Could you check a few things on this model? Use its own coordinates, in mm. A direction names the side the tool comes from. Coordinates: 2 decimals unless noted, no trailing zeros. Loops run counter-clockwise (first coordinate to the right, second up) from the corner with the lowest first, then second, coordinate; pieces in that order, holes last. Notation, with made-up numbers: M -1,61 L 54,61 A10 cw 54,72 Z; hole C 11,71 d2. An arc over 180 degrees is marked long. Write each question's results on one line, items separated by ' | '.
```python
from build123d import *

# Parameters (mm, degrees)
F0_W     = 495.3
F0_H     = 495.3
F1_DEPTH = 838.2
F3_DEPTH = 38.1
F5_DEPTH = 38.1
F7_DEPTH = 1117.6
F9_DEPTH = 127


with BuildPart() as f1:
    # F0 (on Top) → F1 (new body)
    with BuildSketch(Plane.XY):
        Rectangle(F0_W, F0_H)
    extrude(amount=F1_DEPTH)

    # F2 (on face) → F3 (join)
    with BuildSketch(Plane.XZ.offset(247.65)):
        with BuildLine():
            ThreePointArc((0, 273.05), (-68.2625, 204.7875), (0, 136.525))
            Line((0, 136.525), (0, 273.05))
        make_face()
        with BuildLine():
            Line((0, 273.05), (0, 136.525))
            ThreePointArc((0, 136.525), (48.268877, 156.518623), (68.2625, 204.7875))
            ThreePointArc((68.2625, 204.7875), (48.268877, 253.056377), (0, 273.05))
        make_face()
    extrude(amount=F3_DEPTH)

    # F4 (on face) → F5 (join)
    with BuildSketch(Plane.XY.offset(838.2)):
        Polygon((-558.8, 377.825), (-558.8, -247.65), (-558.8, -307.975), (558.8, -307.975), (558.8, -247.65), (558.8, 377.825), align=None)
    extrude(amount=F5_DEPTH)

    # F6 (on face) → F7 (join)
    with BuildSketch(Plane.YZ.offset(558.8)):
        Polygon((-307.975, 838.2), (-307.975, 876.3), (-314.325, 876.3), (-314.325, 820.7375), (-358.775, 820.7375), (-358.775, 814.3875), (-307.975, 814.3875), align=None)
    extrude(amount=-F7_DEPTH)

    # F8 (on face) → F9 (join)
    with BuildSketch(Plane(origin=(0, 0, 0), x_dir=(1, 0, 0), z_dir=(0, 0, -1))):
        Polygon((234.95, 247.65), (247.65, 247.65), (247.65, 431.8), (-247.65, 431.8), (-247.65, 247.65), (-234.95, 247.65), (-234.95, 419.1), (234.95, 419.1), align=None)
    extrude(amount=-F9_DEPTH)


solid = f1.part
```
(1) Imagine slicing it at D-D, the plane z = 789. List the corners of the cut face in (x, y) for me.
Reported:
outline: M -247.65,-247.65 L 247.65,-247.65 L 247.65,247.65 L -247.65,247.65 Z
(2) Imagine slicing it at C-C, the plane x = 374. List the corners of the cut face in (y, z) for me (1 decimal), and give its area (3 significant figures).
Reported:
outline: M -358.8,814.4 L -308,814.4 L -308,838.2 L 377.8,838.2 L 377.8,876.3 L -314.3,876.3 L -314.3,820.7 L -358.8,820.7 Z | area: 26,800 mm2
(3) Which directions (+Z, -Z, +X, -X, +Y, -Y) give clear straight access to the entire face, cutting with the end or side of a thin tool? Please do faces 4 (the flat face through (-1, -285.75, 206)), 5 (the flat face through (-20, -422, 127)), 6 (the flat face through (8, -314.325, 849)).
Reported:
face 4: -Z, +X, -X, -Y | face 5: +X, -X, -Y | face 6: +Z, +X, -X, -Y
(4) If we mould it in two halves opening along X, with no side actions, what happens to faces 1 (the flat face through (8, 37, 876.3)), 2 (the flat face through (-247.65, -21, 413)), 3 (the flat face through (-3, -419.1, 63))? For each: released by +X, released by -X, zero draft, split by the parting line, or undercut.
Reported:
face 1: zero draft | face 2: released by -X | face 3: undercut
(5) Imagine slicing it at B-B, the plane y = 6. List the corners of the cut face in (x, z) for me, and give its area (3 significant figures).
Reported:
outline: M -558.8,838.2 L -247.65,838.2 L -247.65,0 L 247.65,0 L 247.65,838.2 L 558.8,838.2 L 558.8,876.3 L -558.8,876.3 Z | area: 458,000 mm2
(6) Please list where these lines run through material, in increasing order: probe 1 along X at (y, z) = (-326, 70.5); probe 2 along X at (y, z) = (-142.5, 299.5); probe 3 along Z at (x, y) = (-122, -311.5). Write a range as from..to.
Reported:
probe 1: x = -247.65..-234.95, 234.95..247.65 | probe 2: x = -247.65..247.65 | probe 3: z = 814.39..876.3
(7) Will these pins go through, and if not, where does the flat tip stop? P1, Ø3, axis at x = -428, y = -304.5, coming from the -Z side; P2, Ø10, axis at x = 135, z = 376.5, coming from the -Y side; P3, Ø12, axis at x = 83.5, z = 294, coming from the +Y side.
Reported:
P1: stops at z = 838.2 | P2: stops at y = -247.65 | P3: stops at y = 247.65
